from build123d import *

# Parameters (mm, degrees)
F2_R      = 1.5
F3_DEPTH  = 10
F2_R_2    = 2.75
F3_FACE_R = 1.5
F4_DEPTH  = 3
F5_SIZE   = 0.3
F7_DEPTH  = 1.3


with BuildPart() as f3:
    # F2 (on Top) → F3 (new body)
    with BuildSketch(Plane.XY):
        Circle(F2_R)
    extrude(amount=-F3_DEPTH)

    # F2 (on Top) + F3_face (on face) → F4 (join)
    with BuildSketch(Plane.XY):
        Circle(F2_R_2)
        Circle(F2_R, mode=Mode.SUBTRACT)
    with BuildSketch(Plane.XY):
        Circle(F3_FACE_R)
    extrude(amount=F4_DEPTH)

    # F5
    f5_edges = [f3.edges().sort_by_distance(p)[0] for p in [
        (-1.5, 0, -10),
        (-2.75, 0, 3),
    ]]
    chamfer(f5_edges, length=F5_SIZE)

    # F6 (on face) → F7 (cut)
    with BuildSketch(Plane.XY.offset(3)):
        Polygon((1.25, -0.7216878365), (1.25, 0.7216878365), (0, 1.443375673), (-1.25, 0.7216878365), (-1.25, -0.7216878365), (0, -1.443375673), align=None)
    extrude(amount=-F7_DEPTH, mode=Mode.SUBTRACT)


solid = f3.part
For this review, take the finished solid that the model builds, in its own axes (mm). A direction names the side the tool comes from. Round coordinates to 2 decimals unless told otherwise and drop trailing zeros. Write each loop counter-clockwise with the first axis right and the second up, starting at its lowest first coordinate (ties: lowest second). Pieces come first, ordered by that corner, then holes. Notation, with made-up numbers: M -14,79 L -10,79 A8 cw -10,90 Z; hole C 32.25,1.25 d4. An arc over 180 degrees is marked long. Write item = value, one per line. Start each with the question number.
(1) For faces 1 (the face through (-1.25, 0, 2)), 2 (the face through (-1.5, 0.07, -4.78)), 3 (the face through (1.1, -1.1, 3)), list the 3-axis set-ups (+Z, -Z, +X, -X, +Y, -Y) from which the entire face can be reached by the end or side of a thin tool; tool diameter is ignored.
(2) The part is to be moulded in two halves that separate along X. For faces 4 (the face through (1.2, -1.2, 0)), 5 (the face through (-0.596, -2.685, 1.331)), 6 (the face through (-0.616, 1.088, 2.359)), say which applies: +X half, -X half, draft (parallel to the pull), parting line (faces both ways), or undercut.
(3) We need section A-A (y = 0). Give the boundary of the cut face in (x, z).
(4) Clearance check with a flat-ended pin moving along its axis: pin 1 Ø2 at (x, z) = (1.5, -7.5) entering from -Y. State where the tip first meets the part, or that it passes through.
(5) For line 1 along Z through (x, y) = (-1.65, 1.4); line 2 along X through (y, z) = (0.4, -3.25); line 3 along Y through (x, z) = (-0.6, 2), list the stretches that pass through material, from the lowest coordinate up.
(6) We need section B-B (z = 0.5). Give the boundary of the cut face in (x, y).
Results found:
q1.face_1 = +Z
q1.face_2 = -Z
q1.face_3 = +Z, +X, -X, +Y, -Y
q2.face_4 = draft
q2.face_5 = parting line
q2.face_6 = undercut
q3.outline = M -2.75,0 L -1.5,0 L -1.5,-9.7 L -1.2,-10 L 1.2,-10 L 1.5,-9.7 L 1.5,0 L 2.75,0 L 2.75,2.7 L 2.45,3 L 1.25,3 L 1.25,1.7 L -1.25,1.7 L -1.25,3 L -2.45,3 L -2.75,2.7 Z
q4.pin_1 = -1.41
q5.line_1 = 0 to 3
q5.line_2 = -1.45 to 1.45
q5.line_3 = -2.68 to -1.1, 1.1 to 2.68
q6.outline = C 0,0 d5.5
